Model file for the job. Use its own axes, mm. A direction names the side the tool comes from. Give positions to 0.01 mm unless a question says otherwise; leave off trailing zeros. Write each loop counter-clockwise with the first axis right and the second up, starting at its lowest first coordinate (ties: lowest second). Pieces come first, ordered by that corner, then holes.
```python
from build123d import *

# Parameters (mm, degrees)
F0_W      = 72.0000043511
F0_H      = 72.9000046849
F1_DEPTH  = 57.7
F2_W      = 47.4000014365
F2_H      = 48.9999987185
F3_DEPTH  = 49
F4_W      = 12.3000014573
F4_H      = 48.9999987185
F5_DEPTH  = 49
F6_W      = 12.3000014573
F6_H      = 49.0666516125
F7_DEPTH  = 49
F8_W      = 47.4963821471
F8_H      = 11.9500029832
F9_DEPTH  = 49
F10_W     = 46.0287183523
F10_H     = 11.9500029832
F11_DEPTH = 49
F12_R     = 1
F13_R     = 1
F14_R     = 1
F15_R     = 1


with BuildPart() as f1:
    # F0 (on Top) → F1 (new body)
    with BuildSketch(Plane.XY):
        Rectangle(F0_W, F0_H)
    extrude(amount=F1_DEPTH)

    # F2 (on face) → F3 (cut)
    with BuildSketch(Plane(origin=(0, 0, 0), x_dir=(1, 0, 0), z_dir=(0, 0, -1))):
        Rectangle(F2_W, F2_H)
    extrude(amount=-F3_DEPTH, mode=Mode.SUBTRACT)

    # F4 (on face) → F5 (cut)
    with BuildSketch(Plane(origin=(0, 0, 0), x_dir=(1, 0, 0), z_dir=(0, 0, -1))):
        with Locations((-29.8500014469, 0)):
            Rectangle(F4_W, F4_H)
    extrude(amount=-F5_DEPTH, mode=Mode.SUBTRACT)

    # F6 (on face) → F7 (cut)
    with BuildSketch(Plane(origin=(0, 0, 0), x_dir=(1, 0, 0), z_dir=(0, 0, -1))):
        with Locations((29.8500014469, -0.033326447)):
            Rectangle(F6_W, F6_H)
    extrude(amount=-F7_DEPTH, mode=Mode.SUBTRACT)

    # F8 (on face) → F9 (cut)
    with BuildSketch(Plane(origin=(0, 0, 0), x_dir=(1, 0, 0), z_dir=(0, 0, -1))):
        with Locations((-0.0481903553, -30.4750008509)):
            Rectangle(F8_W, F8_H)
    extrude(amount=-F9_DEPTH, mode=Mode.SUBTRACT)

    # F10 (on face) → F11 (cut)
    with BuildSketch(Plane(origin=(0, 0, 0), x_dir=(1, 0, 0), z_dir=(0, 0, -1))):
        with Locations((-0.2511702478, 30.4750008509)):
            Rectangle(F10_W, F10_H)
    extrude(amount=-F11_DEPTH, mode=Mode.SUBTRACT)

    # F12
    f12_edges = [f1.edges().sort_by_distance(p)[0] for p in [
        (0, -36.450002, 57.7),
    ]]
    fillet(f12_edges, radius=F12_R)

    # F13
    f13_edges = [f1.edges().sort_by_distance(p)[0] for p in [
        (-36.000002, 0.5, 57.7),
    ]]
    fillet(f13_edges, radius=F13_R)

    # F14
    f14_edges = [f1.edges().sort_by_distance(p)[0] for p in [
        (0.5, 36.450002, 57.7),
    ]]
    fillet(f14_edges, radius=F14_R)

    # F15
    f15_edges = [f1.edges().sort_by_distance(p)[0] for p in [
        (36.000002, 0, 57.7),
    ]]
    fillet(f15_edges, radius=F15_R)


solid = f1.part
```
1. Probe probe 1 along Y at (x, z) = (-24.5, 22.5); probe 2 along X at (y, z) = (-30.5, 13.5); probe 3 along Y at (x, z) = (23.5, 29). List the from-to ranges inside material, lowest first.
Calculated:
probe 1: y = -36.45 to -24.5, 24.5 to 36.45
probe 2: x = -36 to -23.27, 22.76 to 36
probe 3: y = -36.45 to -24.5
2. Which spindle directions (+Z, -Z, +X, -X, +Y, -Y) get a long thin tool onto all of the face, cutting with end or side? Do faces 4 (the flat face through (-30, -24.5, 24)), 5 (the flat face through (22.763, -30, 24)), 6 (the flat face through (23.7, 31, 24)), 7 (the flat face through (36, -0.2, 49.2)). Say none if no direction does.
Calculated:
face 4: -Z, +X, -X
face 5: -Z, +Y, -Y
face 6: -Z, +Y
face 7: +Z, -Z, +X, +Y, -Y
3. Slice it at A-A, the plane z = 36.5. Write the cut outline in (x, y).
Calculated:
outline: (-36, -35.45) arc R1 ccw to (-35, -36.45) - (-23.27, -36.45) - (-23.27, -24.5) - (-36, -24.5) - close; (-36, 24.5) - (-23.8, 24.5) - (-23.8, 36.45) - (-35, 36.45) arc R1 ccw to (-36, 35.45) - close; (22.76, -36.45) - (35, -36.45) arc R1 ccw to (36, -35.45) - (36, -24.5) - (22.76, -24.5) - close; (23.7, 24.57) - (36, 24.57) - (36, 35.45) arc R1 ccw to (35, 36.45) - (23.7, 36.45) - close
4. Slice it at B-B, the plane y = -28. Write the cut outline in (x, z).
Calculated:
outline: (-36, 0) - (-23.27, 0) - (-23.27, 49) - (22.76, 49) - (22.76, 0) - (36, 0) - (36, 56.7) arc R1 ccw to (35, 57.7) - (-35, 57.7) arc R1 ccw to (-36, 56.7) - close
5. Pin check, flat tips, straight feed: P1, Ø4, axis at y = -21, z = 8, coming from the +X side; P2, Ø8, axis at x = 19.5, z = 30, coming from the +Y side; P3, Ø10, axis at y = 20.5, z = 16.5, coming from the -X side; P4, Ø3, axis at x = -17.5, y = 16, coming from the -Z side. Stop position of each tip, or through.
Calculated:
P1: passes through
P2: stops at y = -24.5
P3: stops at x = -36
P4: stops at z = 49
6. Slice it at D-D, the plane y = -8. Write the cut outline in (x, z).
Calculated:
outline: (-36, 49) - (36, 49) - (36, 56.7) arc R1 ccw to (35, 57.7) - (-35, 57.7) arc R1 ccw to (-36, 56.7) - close
7. Pull direction Y, two halves, no side cores. Call faces 1 (the flat face through (-23.266, -30, 24)), 2 (the flat face through (30, 24.567, 24)), 3 (the flat face through (-24, 36.45, 34)): +Y half, -Y half, draft (parallel to the pull), parting line (faces both ways), or undercut.
Calculated:
face 1: draft
face 2: undercut
face 3: +Y half
8. Slice it at C-C, the plane x = -30. Write the cut outline in (y, z), and give its area (3 significant figures).
Calculated:
outline: (-36.45, 0) - (-24.5, 0) - (-24.5, 49) - (24.5, 49) - (24.5, 0) - (36.45, 0) - (36.45, 56.7) arc R1 ccw to (35.45, 57.7) - (-35.45, 57.7) arc R1 ccw to (-36.45, 56.7) - close
area: 1,800 mm2
